Input: part model. Units: mm. Frame: model coordinates. A direction names the side the tool comes from. Round coordinates to 2 decimals unless told otherwise and drop trailing zeros. Order: outer loops, then holes, each group sorted by start corner. A loop starts at its lowest first (then second) coordinate and runs counter-clockwise, first axis right, second up. Notation, with made-up numbers: M -30,-5.75 L 13,-5.75 A12 cw 13,17.25 Z; hole C -36,70 d11. An arc over 180 degrees is marked long. One line per question, with ' | ' between items.
```python
from build123d import *

# Parameters (mm, degrees)
BOSS_EXTRUDE1_DEPTH = 82.55
CUT_EXTRUDE1_REACH  = 27.4
SKETCH2_R           = 14.2875
CUT_EXTRUDE2_REACH  = 5.175
SKETCH3_W           = 3.175
SKETCH3_H           = 22.225


with BuildPart() as part:
    # Sketch1 → Boss-Extrude1 (new body)
    with BuildSketch(Plane.XY):
        Polygon((47.625, 3.175), (47.625, 25.4), (50.8, 25.4), (50.8, 0), (0, 0), (0, 25.4), (3.175, 25.4), (3.175, 3.175), align=None)
    extrude(amount=BOSS_EXTRUDE1_DEPTH)

    # Sketch2 → Cut-Extrude1 (cut, up to next)
    with BuildSketch(Plane.XZ, mode=Mode.PRIVATE) as cut_extrude1_sk1:
        with Locations((25.4, 50.8)):
            Circle(SKETCH2_R)
    cut_extrude1_tool1 = extrude(cut_extrude1_sk1.sketch, amount=-CUT_EXTRUDE1_REACH, mode=Mode.PRIVATE) & part.part
    add(cut_extrude1_tool1.solids().sort_by_distance((25.4, 0, 50.8))[0], mode=Mode.SUBTRACT)

    # Sketch3 → Cut-Extrude2 (cut, up to next)
    with BuildSketch(Plane(origin=(0, 3.175, 0), x_dir=(1, 0, 0), z_dir=(0, 1, 0)), mode=Mode.PRIVATE) as cut_extrude2_sk1:
        with Locations((46.0375, -11.1125)):
            Rectangle(SKETCH3_W, SKETCH3_H)
    cut_extrude2_tool1 = extrude(cut_extrude2_sk1.sketch, amount=-CUT_EXTRUDE2_REACH, mode=Mode.PRIVATE) & part.part
    add(cut_extrude2_tool1.solids().sort_by_distance((46.0375, 3.175, 11.1125))[0], mode=Mode.SUBTRACT)


solid = part.part
```
Item 1: Section query C-C, the plane y = 4. Return loops of the section in (x, z) (3 decimals).
Report:
outline: M 0,0 L 3.175,0 L 3.175,82.55 L 0,82.55 Z; M 47.625,0 L 50.8,0 L 50.8,82.55 L 47.625,82.55 Z
Item 2: Access query for faces 4 (the flat face through (46, 2, 22.225)), 5 (the flat face through (24, 2, 82.55)), 6 (the flat face through (25, 3.175, 32)). Directions: +Z, -Z, +X, -X, +Y, -Y. A direction counts if a zero-diameter tool reaches every point of the face in a straight line with its end or side. Return the directions, or none.
Report:
face 4: -Z, +Y, -Y | face 5: +Z, +X, -X, +Y, -Y | face 6: +Z, -Z, +Y
Item 3: Mould query, pull axis X, two halves, no side actions, for faces 1 (the flat face through (3.175, 14, 41)), 2 (the flat face through (49, 25.4, 41)), 3 (the flat face through (0, 13, 41)). Classes: +X half, -X half, draft (parallel to the pull), parting line (faces both ways), or undercut.
Report:
face 1: undercut | face 2: draft | face 3: -X half
Item 4: Line query: line 1 along X through (y, z) = (8, 17.5) (3 decimals); line 2 along Z through (x, y) = (25.4, 1.65); line 3 along Z through (x, y) = (24, 3). Output: solid intervals per line, ascending. Write a range as from..to.
Report:
line 1: 0..3.175, 47.625..50.8 | line 2: 0..36.51, 65.09..82.55 | line 3: 0..36.58, 65.02..82.55
Item 5: Section query D-D, the plane z = 50.8. Return loops of the section in (x, y) (1 decimal).
Report:
outline: M 0,0 L 11.1,0 L 11.1,3.2 L 3.2,3.2 L 3.2,25.4 L 0,25.4 Z; M 39.7,0 L 50.8,0 L 50.8,25.4 L 47.6,25.4 L 47.6,3.2 L 39.7,3.2 Z
Item 6: Section query A-A, the plane z = 15. Return loops of the section in (x, y) (3 decimals), plus the area to 3 significant figures.
Report:
outline: M 0,0 L 44.45,0 L 44.45,3.175 L 3.175,3.175 L 3.175,25.4 L 0,25.4 Z; M 47.625,0 L 50.8,0 L 50.8,25.4 L 47.625,25.4 Z | area: 292 mm²
Item 7: First-contact query: pin 1 (1 mm diameter, centred on x = 46, y = 1, fed in from -Z) (3 decimals); pin 2 (1 mm diameter, centred on x = 31.5, z = 13, fed in from +Y) (3 decimals). Flat tips, straight axial feed; report the tip coordinate or a pass-through.
Report:
pin 1: z = 22.225 | pin 2: y = 3.175
